from build123d import *

# Parameters (mm, degrees)
SKETCH_W     = 1226
SKETCH_H     = 690
PAD_DEPTH    = 60
SKETCH001_W  = 1178.222099
SKETCH001_H  = 634.606854
POCKET_DEPTH = 5
SKETCH002_W  = 697.600952
SKETCH002_H  = 639.273081
PAD001_DEPTH = 20
PAD002_DEPTH = 20


with BuildPart() as part:
    # Sketch → Pad (new body)
    with BuildSketch(Plane.YZ):
        with Locations((613, 345)):
            Rectangle(SKETCH_W, SKETCH_H)
    extrude(amount=PAD_DEPTH)

    # Sketch001 (on Face6 of Pad) → Pocket (cut)
    with BuildSketch(Plane.YZ.offset(60)):
        with Locations((610.844516, 346.005472)):
            Rectangle(SKETCH001_W, SKETCH001_H)
    extrude(amount=-POCKET_DEPTH, mode=Mode.SUBTRACT)

    # Sketch002 (on Face4 of Pocket) → Pad001 (join)
    with BuildSketch(Plane(origin=(0, 0, 0), x_dir=(0, 1, 0), z_dir=(-1, 0, 0))):
        with Locations((619.926025, -343.598201)):
            Rectangle(SKETCH002_W, SKETCH002_H)
    extrude(amount=PAD001_DEPTH)

    # Sketch003 (on Face1 of Pad001) → Pad002 (join)
    with BuildSketch(Plane.YX):
        Polygon((87.634308, -42.883045), (29.457521, 98.781487), (45.932869, 105.38868), (106.168274, -33.616066), align=None)
        Polygon((1123.258545, -38.812469), (1166.333008, 103.550873), (1181.619751, 100.072845), (1138.033447, -42.506088), align=None)
    extrude(amount=PAD002_DEPTH)


solid = part.part
Source: CAD feature listing. Evaluate the final solid. Frame: model axes, mm. A direction names the side the tool comes from. Give positions to 0.01 mm unless a question says otherwise; leave off trailing zeros. Write each loop counter-clockwise with the first axis right and the second up, starting at its lowest first coordinate (ties: lowest second). Pieces come first, ordered by that corner, then holes. Notation, with made-up numbers: M -18.5,58.25 L -5.5,58.25 A13 ccw -5.5,75.25 Z; hole C 29.5,17.5 d5. An arc over 180 degrees is marked long. Return JSON: item names as keys, results as strings. Group by question number.
1) Cut plane A-A, the plane y = 286.5. Output: boundary loops of the cut face in (x, z), plus the area to 3 significant figures.
2) Cut plane C-C, the plane z = 390. Output: boundary loops of the cut face in (x, y), plus the area to 3 significant figures.
3) Set-up query: faces 4 (the face through (-21, 88, 0)), 5 (the face through (82, 1168, 0)), 6 (the face through (30, 27, 0)), 7 (the face through (30, 1196, 0)). Return all of +Z, -Z, +X, -X, +Y, -Y with unobstructed straight access to the full face (end or side cutting, diameter ignored); none if empty.
4) Pin query (flat end, axial travel): P1, Ø22, axis at x = -32, y = 1138, coming from the +Z side; P2, Ø10, axis at x = -5.5, y = 671.5, coming from the -Z side; P3, Ø5, axis at y = 511, z = 369.5, coming from the -X side. Return the tip coordinate at first contact, or that it passes through.
5) Pull-direction query (Z, two-part tool) for faces 1 (the face through (55, 603, 350)), 2 (the face through (31.373, 1144.494, -9.86)), 3 (the face through (-21, 1137, 0)); classes: pulls with the +Z half, pulls with the -Z half, needs draft (parallel to the pull), parting line crosses it, or undercut.
6) Material intervals for line 1 along X through (y, z) = (953.5, 23); line 2 along Y through (x, z) = (-17, 432.5); line 3 along Z through (x, y) = (34, 648), sorted ascending. Write a range as [from, to].
7) Cut plane B-B, the plane x = 77. Output: boundary loops of the cut face in (y, z), plus the area to 3 significant figures.
Recorded:
{
 "1": {"outline": "M -20,23.96 L 0,23.96 L 0,0 L 60,0 L 60,28.7 L 55,28.7 L 55,663.31 L 60,663.31 L 60,690 L 0,690 L 0,663.23 L -20,663.23 Z", "area": "51,000 mm²"},
 "2": {"outline": "M -20,271.13 L 0,271.13 L 0,0 L 60,0 L 60,21.73 L 55,21.73 L 55,1199.96 L 60,1199.96 L 60,1226 L 0,1226 L 0,968.73 L -20,968.73 Z", "area": "81,600 mm²"},
 "3": {"face 4": "+Z, -X, +Y, -Y", "face 5": "+Z, +X, +Y, -Y", "face 6": "-Z, -X, -Y", "face 7": "-Z, -X, +Y"},
 "4": {"P1": "stops at z = 0", "P2": "stops at z = 23.96", "P3": "stops at x = -20"},
 "5": {"face 1": "undercut", "face 2": "needs draft", "face 3": "pulls with the +Z half"},
 "6": {"line 1": "x = [0, 60]", "line 2": "y = [271.13, 968.73]", "line 3": "z = [0, 690]"},
 "7": {"outline": "M 38.4,-20 L 58.23,-20 L 58.23,0 L 38.4,0 Z; M 1158.3,-20 L 1174.57,-20 L 1174.57,0 L 1158.3,0 Z", "area": "722 mm²"}
}
